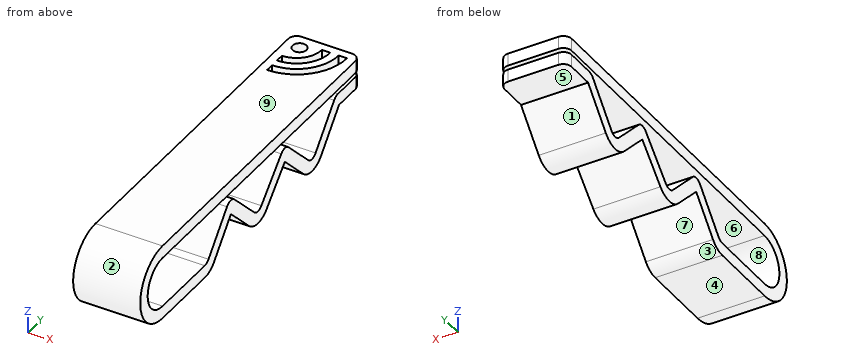
from build123d import *

# Parameters (mm, degrees)
F1_DEPTH = 8
F2_R     = 0.828427
F3_DEPTH = 1.5
F4_R     = 1


with BuildPart() as f1:
    # F0 (on Right) → F1 (new body)
    with BuildSketch(Plane.YZ):
        with BuildLine():
            ThreePointArc((0, -3), (-3, 0), (0, 3))
            Line((0, 3), (40, 3))
            Line((40, 3), (40, 4.5))
            Line((40, 4.5), (0, 4.5))
            ThreePointArc((0, 4.5), (-4.5, 0), (0, -4.5))
            Line((0, -4.5), (8.541805, -4.5))
            ThreePointArc((8.541805, -4.5), (9.583182, -4.272781), (10.435262, -3.632429))
            Line((10.435262, -3.632429), (13.826929, 0.301572))
            Line((13.826929, 0.301572), (17.512715, -3.358312))
            ThreePointArc((17.512715, -3.358312), (19.285663, -4.084296), (21.051901, -3.342136))
            Line((21.051901, -3.342136), (24.728998, 0.376483))
            Line((24.728998, 0.376483), (28.439931, -3.30837))
            ThreePointArc((28.439931, -3.30837), (30.298208, -4.032508), (32.09491, -3.16681))
            Line((32.09491, -3.16681), (35.687292, 1))
            Line((35.687292, 1), (40, 1))
            Line((40, 1), (40, 2.5))
            Line((40, 2.5), (35.458195, 2.5))
            ThreePointArc((35.458195, 2.5), (35.041644, 2.409113), (34.700812, 2.152971))
            Line((34.700812, 2.152971), (30.958836, -2.187352))
            ThreePointArc((30.958836, -2.187352), (30.240155, -2.533632), (29.496844, -2.243977))
            Line((29.496844, -2.243977), (25.430372, 1.793918))
            ThreePointArc((25.430372, 1.793918), (24.721192, 2.084312), (24.014697, 1.787448))
            Line((24.014697, 1.787448), (19.985303, -2.287448))
            ThreePointArc((19.985303, -2.287448), (19.278808, -2.584312), (18.569628, -2.293918))
            Line((18.569628, -2.293918), (14.503156, 1.743977))
            ThreePointArc((14.503156, 1.743977), (13.759845, 2.033632), (13.041164, 1.687352))
            Line((13.041164, 1.687352), (9.299188, -2.652971))
            ThreePointArc((9.299188, -2.652971), (8.958356, -2.909113), (8.541805, -3))
            Line((8.541805, -3), (0, -3))
        make_face()
    extrude(amount=F1_DEPTH)

    # F2 (on face) → F3 (cut, through all)
    with BuildSketch(Plane.XY.offset(4.5)):
        with BuildLine():
            ThreePointArc((4, 39), (3.12132, 36.87868), (1, 36))
            Line((1, 36), (1, 35))
            ThreePointArc((1, 35), (3.828427, 36.171573), (5, 39))
            Line((5, 39), (4, 39))
        make_face()
        with BuildLine():
            ThreePointArc((6, 39), (4.535534, 35.464466), (1, 34))
            Line((1, 34), (1, 33))
            ThreePointArc((1, 33), (5.242641, 34.757359), (7, 39))
            Line((7, 39), (6, 39))
        make_face()
        with Locations((1.828427, 38.171573)):
            Circle(F2_R)
    extrude(amount=-F3_DEPTH, mode=Mode.SUBTRACT)

    # F4
    f4_edges = [f1.edges().sort_by_distance(p)[0] for p in [
        (8, 40, 3.75),
        (8, 40, 1.75),
        (0, 40, 1.75),
        (0, 40, 3.75),
    ]]
    fillet(f4_edges, radius=F4_R)


solid = f1.part
Work out the finished part from the listing and answer in its coordinate system (mm). Face numbers are marked on the shaded views. A direction names the side the tool comes from. Give positions to 0.01 mm unless a question says otherwise; leave off trailing zeros. Loops run counter-clockwise (first coordinate to the right, second up) from the corner with the lowest first, then second, coordinate; pieces in that order, holes last. Notation, with made-up numbers: (46.25, 76.5) -> (96.25, 76.5) arc R24 ccw to (96.25, 87.5) -> close; hole circle Ø2 at (88, 46.25). An arc over 180 degrees is marked (long way). Use a Markdown table: item, result. Add a question column.
1. Determine the mould class of the marked faces 1, 2, 3 and 4 for opening direction Y: released by +Y, released by -Y, zero draft, split by the parting line, or undercut.
2. Section B-B on z = -1.75 is taken. Determine the outline of the cut face in (x, y), and give its area (3 significant figures).
3. For the marked faces 5, 6, 7, 8 and 9, determine the directions among +Z, -Z, +X, -X, +Y, -Y from which every point of the face is accessible in a straight line to the end or side of a thin tool.
4. Section A-A on y = 4.5 is taken. Determine the outline of the cut face in (x, z).
5. Section C-C on y = -1 is taken. Determine the outline of the cut face in (x, z), and give its area (3 significant figures).
6. Flat-ended cylindrical pins translate along their axes: pin 1 Ø4.5 at (x, y) = (5.5, 39) entering from -Z; pin 2 Ø3.5 at (x, y) = (4.5, 37.5) entering from +Z; pin 3 Ø0.5 at (x, z) = (6.5, 3.5) entering from -Y; pin 4 Ø4 at (x, y) = (2.5, 24) entering from -Z. Find the tip coordinate at first contact, or state that the pin passes through.
7. Find the intervals of material crossed by probe 1 along Z at (x, y) = (5.75, 6); probe 2 along Y at (x, z) = (6, 0.75); probe 3 along Z at (x, y) = (0.75, 36), in increasing order.
Results below:
| question | item | result |
|---|---|---|
| 1 | face 1 | released by +Y |
| 1 | face 2 | released by -Y |
| 1 | face 3 | undercut |
| 1 | face 4 | zero draft |
| 2 | outline | (0, -4.15) -> (8, -4.15) -> (8, -2.44) -> (0, -2.44) -> close; (0, 10.08) -> (8, 10.08) -> (8, 12.06) -> (0, 12.06) -> close; (0, 15.89) -> (8, 15.89) -> (8, 18.02) -> (0, 18.02) -> close; (0, 20.52) -> (8, 20.52) -> (8, 22.63) -> (0, 22.63) -> close; (0, 26.87) -> (8, 26.87) -> (8, 29) -> (0, 29) -> close; (0, 31.34) -> (8, 31.34) -> (8, 33.32) -> (0, 33.32) -> close |
| 2 | area | 96.3 mm^2 |
| 3 | face 5 | -Z, +X, -X, +Y |
| 3 | face 6 | +X, -X, +Y |
| 3 | face 7 | -Z, +X, -X |
| 3 | face 8 | +X, -X |
| 3 | face 9 | +Z, +X, -X, +Y, -Y |
| 4 | outline | (0, -4.5) -> (8, -4.5) -> (8, -3) -> (0, -3) -> close; (0, 3) -> (8, 3) -> (8, 4.5) -> (0, 4.5) -> close |
| 5 | outline | (0, -4.39) -> (8, -4.39) -> (8, -2.83) -> (0, -2.83) -> close; (0, 2.83) -> (8, 2.83) -> (8, 4.39) -> (0, 4.39) -> close |
| 5 | area | 24.9 mm^2 |
| 6 | pin 1 | stops at z = 1 |
| 6 | pin 2 | stops at z = 4.5 |
| 6 | pin 3 | stops at y = -3.11 |
| 6 | pin 4 | stops at z = -2.38 |
| 7 | probe 1 | z = -4.5 to -3, 3 to 4.5 |
| 7 | probe 2 | y = -4.44 to -2.9, 12.23 to 15.5, 22.99 to 26.48, 33.49 to 35.47 |
| 7 | probe 3 | z = 1 to 2.5, 3 to 4.5 |
